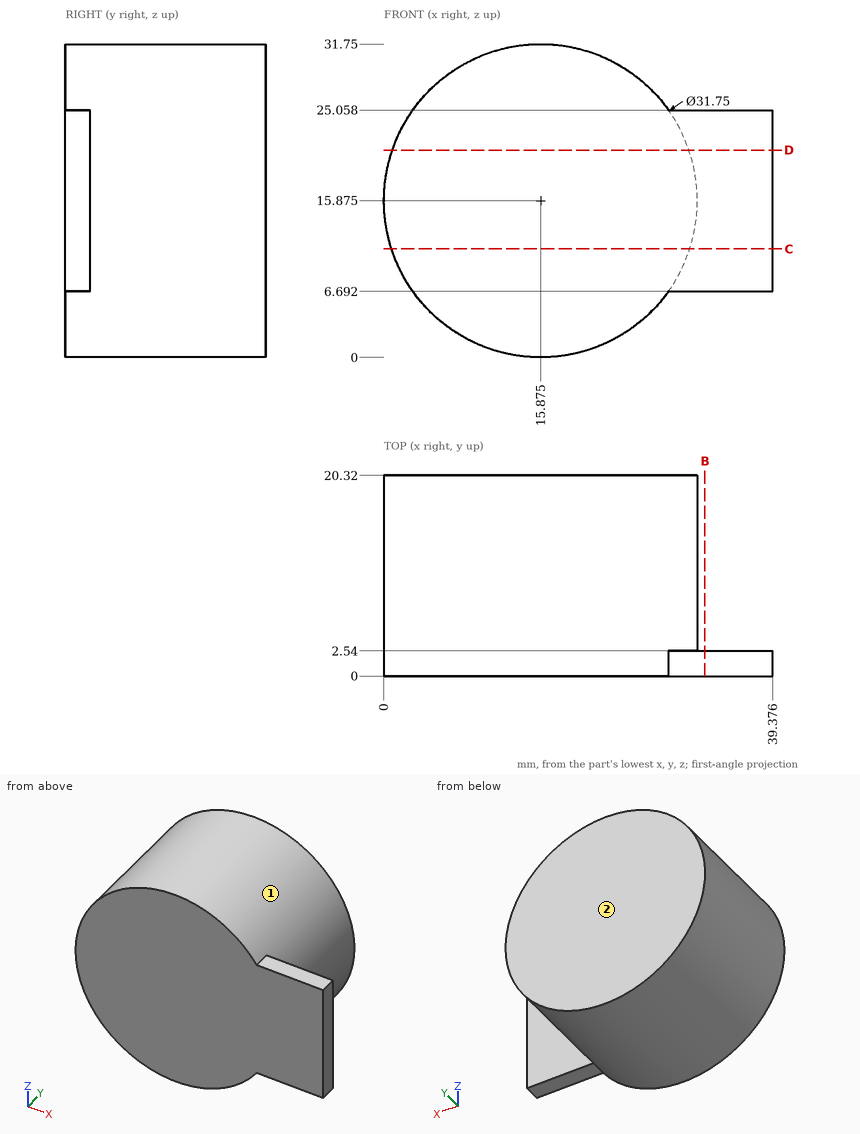
Part print with two shaded views. Sizes in mm from the minimum x, y, z corner. Coordinates: 2 decimals unless noted, no trailing zeros. Order: outer loops, then holes, each group sorted by start corner. A loop starts at its lowest first (then second) coordinate and runs counter-clockwise, first axis right, second up. Notation, with made-up numbers: (74.25, 1) - (123.25, 1) arc R20 ccw to (123.25, 11) - close; hole circle Ø4 at (64.5, 79.5). An arc over 180 degrees is marked (long way). Answer in a Markdown table with one row per item.
1. Slice it at B-B, the plane x = 32.5. List the corners of the cut face in (y, z).
Answer:
| item | result |
|---|---|
| outline | (0, 6.69) - (2.54, 6.69) - (2.54, 25.06) - (0, 25.06) - close |
2. Pull direction Z, two halves, no side cores. Call the marked faces 1 and 2: +Z half, -Z half, draft (parallel to the pull), parting line (faces both ways), or undercut.
Answer:
| item | result |
|---|---|
| face 1 | parting line |
| face 2 | draft |
3. Drill centre lines: L1, parallel to Y at x = 32.5, z = 11.5; L2, parallel to X at y = 15.5, z = 17; L3, parallel to Z at x = 20.5, y = 5. Where is each one in solid material? Low to high. Write a range as from..to.
Answer:
| item | result |
|---|---|
| L1 | 0..2.54 |
| L2 | 0.04..31.71 |
| L3 | 0.69..31.06 |
4. Flat gauge pins, fed straight in: P1, Ø3, axis at y = 4, z = 15.5, coming from the -X side; P2, Ø1.3, axis at x = 32.5, y = 0.5, coming from the +Z side; P3, Ø4, axis at y = 15, z = 19, coming from the +X side; P4, Ø5, axis at y = 10, z = 24, coming from the +X side. Where does each tip first touch, or does it go through?
Answer:
| item | result |
|---|---|
| P1 | x = 0 |
| P2 | z = 25.06 |
| P3 | x = 31.71 |
| P4 | x = 30.72 |
5. Slice it at C-C, the plane z = 11. List the corners of the cut face in (x, y), then the cut area to 3 significant figures.
Answer:
| item | result |
|---|---|
| outline | (0.77, 0) - (39.38, 0) - (39.38, 2.54) - (30.98, 2.54) - (30.98, 20.32) - (0.77, 20.32) - close |
| area | 635 mm² |
6. Slice it at D-D, the plane z = 21. List the corners of the cut face in (x, y), then the cut area to 3 significant figures.
Answer:
| item | result |
|---|---|
| outline | (0.85, 0) - (39.38, 0) - (39.38, 2.54) - (30.9, 2.54) - (30.9, 20.32) - (0.85, 20.32) - close |
| area | 632 mm² |
